Could you check a few things on this drawing? It's one solid part, dimensions in mm from its lowest x, y, z. A direction names the side the tool comes from. Coordinates: 2 decimals unless noted, no trailing zeros. Order: outer loops, then holes, each group sorted by start corner. A loop starts at its lowest first (then second) coordinate and runs counter-clockwise, first axis right, second up. Notation, with made-up numbers: (-5.75, 44) - (18.25, 44) arc R18 ccw to (18.25, 52) - close; hole circle Ø4 at (76.5, 25.25). An arc over 180 degrees is marked (long way). Answer in a Markdown table with one row per item. Add a question column.
Item 1: I want a section at C-C (y = 11.25). Please give me the cut outline in (x, z) (3 decimals).
Item 2: If I drill on line 1 along Y through (x, z) = (1, 1.5); line 2 along Y through (x, z) = (6.75, 1.9); line 3 along X through (y, z) = (9, 2.4), over which ranges is the centre line in solid material (lowest first)? Write a range as from..to.
Item 3: I want a section at A-A (y = 1.75). Please give me the cut outline in (x, z) (3 decimals), plus the area to 3 significant figures.
Item 4: On a 3-axis mill with a long thin cutter (end or side, diameter ignored), from which of +Z, -Z, +X, -X, +Y, -Y can I reach the whole of each face in a straight line? I mean the marked faces 1, 2, 3 and 4. Say none if no direction works.
Item 5: Thinking about a two-plate mould opening in X: for the marked faces 5, 6, 7 and 8, which applies, +X half, -X half, draft (parallel to the pull), parting line (faces both ways), or undercut?
Item 6: I want a section at B-B (x = 1.75). Please give me the cut outline in (y, z) (3 decimals).
Item 7: Will these pins go through, and if not, where does the flat tip stop? pin 1 Ø1.6 at (x, z) = (5.5, 1.5) entering from +Y; pin 2 Ø1.7 at (x, y) = (3, 10) entering from +Z (3 decimals); pin 3 Ø0.5 at (x, y) = (3, 10) entering from -Z (3 decimals).
Item 8: I want a section at D-D (z = 1). Please give me the cut outline in (x, y), plus the area to 3 significant figures.
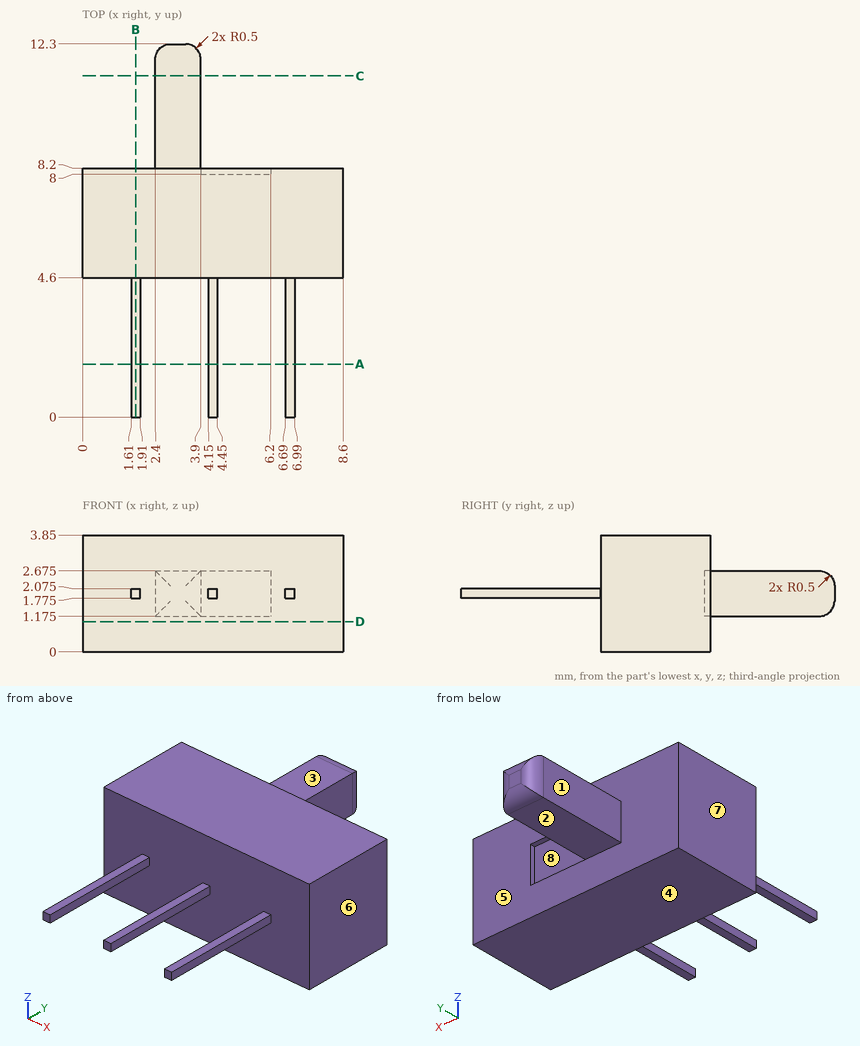
Values follow:
| question | item | result |
|---|---|---|
| 1 | outline | (2.4, 1.175) - (3.9, 1.175) - (3.9, 2.675) - (2.4, 2.675) - close |
| 2 | line 1 | y = 4.6..8.2 |
| 2 | line 2 | y = 0..8.2 |
| 2 | line 3 | x = 2.4..3.9 |
| 3 | outline | (1.61, 1.775) - (1.91, 1.775) - (1.91, 2.075) - (1.61, 2.075) - close; (4.15, 1.775) - (4.45, 1.775) - (4.45, 2.075) - (4.15, 2.075) - close; (6.69, 1.775) - (6.99, 1.775) - (6.99, 2.075) - (6.69, 2.075) - close |
| 3 | area | 0.270 mm^2 |
| 4 | face 1 | +Z, -Z, -X, +Y |
| 4 | face 2 | -Z, +X, -X, +Y |
| 4 | face 3 | +Z, +X, -X, +Y |
| 4 | face 4 | -Z, +X, -X, +Y, -Y |
| 5 | face 5 | draft |
| 5 | face 6 | +X half |
| 5 | face 7 | -X half |
| 5 | face 8 | undercut |
| 6 | outline | (0, 1.775) - (4.6, 1.775) - (4.6, 0) - (8.2, 0) - (8.2, 3.85) - (4.6, 3.85) - (4.6, 2.075) - (0, 2.075) - close |
| 7 | pin 1 | stops at y = 8.2 |
| 7 | pin 2 | stops at z = 2.675 |
| 7 | pin 3 | stops at z = 1.175 |
| 8 | outline | (0, 4.6) - (8.6, 4.6) - (8.6, 8.2) - (0, 8.2) - close |
| 8 | area | 31.0 mm^2 |
